Geometry check sheet. Reference: the model listing, model coordinates, mm. A direction names the side the tool comes from. Coordinates: 2 decimals unless noted, no trailing zeros. Order: outer loops, then holes, each group sorted by start corner. A loop starts at its lowest first (then second) coordinate and runs counter-clockwise, first axis right, second up. Notation, with made-up numbers: (40.5, -4.5) - (62.5, -4.5) arc R28 cw to (62.5, 28.5) - close; hole circle Ø2 at (17.5, -11). An arc over 180 degrees is marked (long way). Return JSON: item names as keys, results as strings. Group by question number.
Item 1: Gauge pin test, flat ends, axial feed: pin 1 (0.8 mm diameter, centred on y = -24.5, z = 31.5, fed in from -X); pin 2 (12 mm diameter, centred on x = -6.5, y = -2.5, fed in from +Z); pin 3 (6 mm diameter, centred on y = -2, z = 15, fed in from -X). Record the tip position at first contact, or that the pin passes through.
Item 2: Tool access check on faces 4 (the flat face through (0, -19, 38.167)), 5 (the flat face through (2, -24, 30.7)), 6 (the flat face through (0, 20, 4)). Record the directions out of +Z, -Z, +X, -X, +Y, -Y that give a thin tool (end or side, any length) a straight path to the whole face; none if there is none.
Item 3: Scan lines: probe 1 along Y at (x, z) = (-5, 29.7); probe 2 along Y at (x, z) = (0, 41.85); probe 3 along X at (y, z) = (-24, 29). Record each from-to range of solid material in increasing order.
Item 4: Section check A-A on x = 5. Give the number of separate pieces and of enclosed holes in the cut face, then the cut area to 3 significant figures.
Item 5: Section check B-B on z = 29.5. Enter the section's corners in (x, y).
Item 6: Draft check along Y on faces 1 (the cylindrical face through (-5.434, 22.798, 29.221)), 2 (the flat face through (0, 27.25, 29)), 3 (the flat face through (9.99, 0, 18)). Enter one of: pulls with the +Y half, pulls with the -Y half, needs draft (parallel to the pull), parting line crosses it, or undercut.
from build123d import *

# Parameters (mm, degrees)
SKETCH1_W                = 40
SKETCH1_H                = 20
BOSS_EXTRUDE1_DEPTH      = 40.5
SKETCH2_W                = 7.25
SKETCH2_H                = 3
BOSS_EXTRUDE2_DEPTH      = 20
SKETCH3_R                = 2
CUT_EXTRUDE1_DEPTH       = 3
SKETCH4_R                = 2.9
SKETCH4_R_2              = 1.45
BOSS_EXTRUDE3_DEPTH      = 5
CUT_EXTRUDE2_DEPTH       = 20
SKETCH5_W                = 20
SKETCH5_H                = 40
SKETCH5_W_2              = 19.98
SKETCH5_H_2              = 39.98
CUT_EXTRUDE3_DEPTH       = 20
BOSS_EXTRUDE5_DEPTH      = 1.3
BOSS_EXTRUDE5_DEPTH_BACK = 1.3


with BuildPart() as part:
    # Sketch1 → Boss-Extrude1 (new body)
    with BuildSketch(Plane(origin=(0, 0, 0), x_dir=(0, 1, 0), z_dir=(0, 0, 1))):
        Rectangle(SKETCH1_W, SKETCH1_H)
    extrude(amount=BOSS_EXTRUDE1_DEPTH)

    # Sketch2 → Boss-Extrude2 (add)
    with BuildSketch(Plane.YZ.offset(10)):
        with Locations((-23.625, 29.2)):
            Rectangle(SKETCH2_W, SKETCH2_H)
        with Locations((23.625, 29.2)):
            Rectangle(SKETCH2_W, SKETCH2_H)
        Polygon((20, 38.166547622), (13.826265312, 40.5), (20, 40.5), align=None)
        Polygon((-20, 38.166547622), (-17.798587441, 38.166547622), (-15.465135063, 40.5), (-20, 40.5), align=None)
    extrude(amount=-BOSS_EXTRUDE2_DEPTH)

    # Sketch3 → Cut-Extrude1 (cut)
    with BuildSketch(Plane.XY.offset(30.7)):
        with Locations((-5, 24.75)):
            Circle(SKETCH3_R)
        with Locations((5, 24.75)):
            Circle(SKETCH3_R)
        with Locations((-5, -24.75)):
            Circle(SKETCH3_R)
        with Locations((5, -24.75)):
            Circle(SKETCH3_R)
    extrude(amount=-CUT_EXTRUDE1_DEPTH, mode=Mode.SUBTRACT)

    # Sketch4 → Boss-Extrude3 (add)
    with BuildSketch(Plane.XY.offset(40.5)):
        with Locations((0, -10)):
            Circle(SKETCH4_R)
        with Locations((0, -10)):
            Circle(SKETCH4_R_2, mode=Mode.SUBTRACT)
    extrude(amount=BOSS_EXTRUDE3_DEPTH)

    # Sketch2<2> → Cut-Extrude2 (cut)
    with BuildSketch(Plane.YZ.offset(10)):
        Polygon((-20, 40.5), (-20, 38.166547622), (-17.798587441, 38.166547622), (-15.465135063, 40.5), align=None)
        Polygon((20, 40.5), (13.826265312, 40.5), (20, 38.166547622), align=None)
    extrude(amount=-CUT_EXTRUDE2_DEPTH, mode=Mode.SUBTRACT)

    # Sketch5 → Cut-Extrude3 (cut)
    with BuildSketch(Plane(origin=(0, 0, 27.7), x_dir=(1, 0, 0), z_dir=(0, 0, -1))):
        Rectangle(SKETCH5_W, SKETCH5_H)
        Rectangle(SKETCH5_W_2, SKETCH5_H_2, mode=Mode.SUBTRACT)
    extrude(amount=CUT_EXTRUDE3_DEPTH, mode=Mode.SUBTRACT)

    # Sketch6 → Boss-Extrude5 (add, two sides: drawn at the far end of the back side and taken through both)
    with BuildSketch(Plane.YZ.offset(-BOSS_EXTRUDE5_DEPTH_BACK)):
        Polygon((-26.65, 30.7), (-20, 32.2), (-20, 30.7), align=None)
        Polygon((20, 32.2), (26.65, 30.7), (20, 30.7), align=None)
    extrude(amount=BOSS_EXTRUDE5_DEPTH + BOSS_EXTRUDE5_DEPTH_BACK)


solid = part.part
Computed:
{
 "1": {"pin 1": "stops at x = -1.3", "pin 2": "stops at z = 40.5", "pin 3": "stops at x = -9.99"},
 "2": {"face 4": "+Z, +X, -X, -Y", "face 5": "+Z, -Y", "face 6": "-Z, +X, -X, +Y"},
 "3": {"probe 1": "y = -27.25 to -26.75, -22.75 to 22.75, 26.75 to 27.25", "probe 2": "y = -12.9 to -11.45, -8.55 to -7.1", "probe 3": "x = -10 to -6.85, -3.15 to 3.15, 6.85 to 10"},
 "4": {"separate pieces": "3", "enclosed holes": "0", "area": "1,620 mm²"},
 "5": {"outline": "(-10, -27.25) - (10, -27.25) - (10, 27.25) - (-10, 27.25) - close; hole circle Ø4 at (-5, -24.75); hole circle Ø4 at (-5, 24.75); hole circle Ø4 at (5, -24.75); hole circle Ø4 at (5, 24.75)"},
 "6": {"face 1": "undercut", "face 2": "pulls with the +Y half", "face 3": "needs draft"}
}
